Could you check a few things on this drawing? It's one solid part, dimensions in mm from its lowest x, y, z. Give positions to 0.01 mm unless a question says otherwise; leave off trailing zeros. Loops run counter-clockwise (first coordinate to the right, second up) from the corner with the lowest first, then second, coordinate; pieces in that order, holes last. Notation, with made-up numbers: (77, 47.5) - (131, 47.5) arc R9 ccw to (131, 56.5) - close; hole circle Ø8 at (2, 31.25). An arc over 180 degrees is marked (long way). Write each question's results on one line, items separated by ' | '. Start each with the question number.
(1) I need wall thicknesses on line 1 (Z direction, x = 26, y = 21.5); line 2 (Y direction, x = 21.5, z = 7.25) (1 decimal); line 3 (Y direction, x = 50, z = 2.5). Which ranges of each line are inside material? Lowest first, please.
(2) Suppose I cut it at D-D (z = 14.75). Please give me the cut outline in (x, y).
(3) Suppose I cut it at A-A (x = 36.83). Please give me the cut outline in (y, z).
(4) Suppose I cut it at B-B (y = 33.02). Please give me the cut outline in (x, z), and give its area (3 significant figures).
(5) For pin 1 (2 mm diameter, centred on x = 3, z = 1.5, fed in from -Y); pin 2 (2 mm diameter, centred on x = 7.5, y = 15, fed in from -Z); pin 3 (5 mm diameter, centred on x = 37, z = 13, fed in from +Y); pin 4 (1 mm diameter, centred on x = 62, z = 2.5, fed in from -Y), each with a flat end and sliding along its axis, tell me the tip position at first contact or that it passes through.
(6) If we mould it in two halves opening along Y, with no side actions, what happens to the marked faces 1, 2 and 3? For each: released by +Y, released by -Y, zero draft, split by the parting line, or undercut.
(7) Suppose I cut it at C-C (z = 3.75). Please give me the cut outline in (x, y).
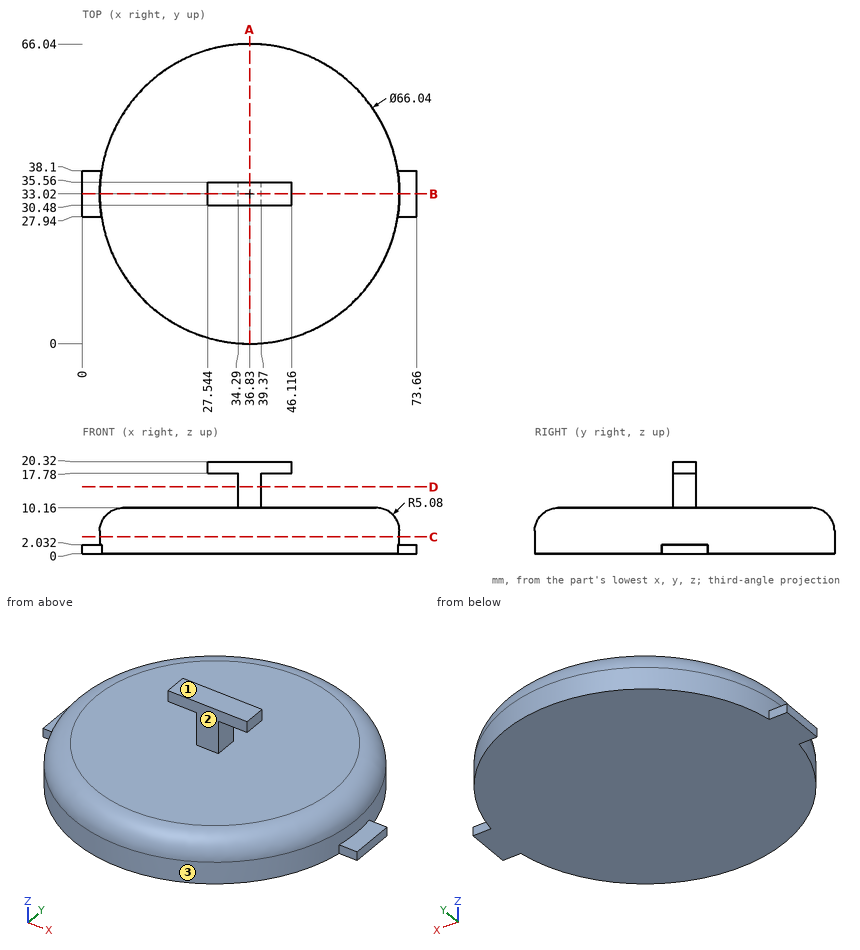
Output values:
1) line 1: 0 to 10.16 | line 2: 4.3 to 61.7 | line 3: 2.74 to 63.3
2) outline: (34.29, 30.48) - (39.37, 30.48) - (39.37, 35.56) - (34.29, 35.56) - close
3) outline: (0, 0) - (66.04, 0) - (66.04, 5.08) arc R5.08 ccw to (60.96, 10.16) - (35.56, 10.16) - (35.56, 20.32) - (30.48, 20.32) - (30.48, 10.16) - (5.08, 10.16) arc R5.08 ccw to (0, 5.08) - close
4) outline: (0, 0) - (73.66, 0) - (73.66, 2.03) - (69.85, 2.03) - (69.85, 5.08) arc R5.08 ccw to (64.77, 10.16) - (39.37, 10.16) - (39.37, 17.78) - (46.12, 17.78) - (46.12, 20.32) - (27.54, 20.32) - (27.54, 17.78) - (34.29, 17.78) - (34.29, 10.16) - (8.89, 10.16) arc R5.08 ccw to (3.81, 5.08) - (3.81, 2.03) - (0, 2.03) - close | area: 761 mm2
5) pin 1: y = 27.94 | pin 2: through | pin 3: y = 35.56 | pin 4: y = 11.07
6) face 1: zero draft | face 2: released by -Y | face 3: split by the parting line
7) outline: circle Ø66.04 at (36.83, 33.02)
